Geometry check sheet. Reference: drawing and pictorial views, mm from the part's lowest x, y, z. A direction names the side the tool comes from. Round coordinates to 2 decimals unless told otherwise and drop trailing zeros. Write each loop counter-clockwise with the first axis right and the second up, starting at its lowest first coordinate (ties: lowest second). Pieces come first, ordered by that corner, then holes. Notation, with made-up numbers: (4, 69) -> (63, 69) arc R21 ccw to (63, 80) -> close; hole circle Ø8 at (39.5, 78.5). An arc over 180 degrees is marked (long way). Answer as a JSON object with one key per item and string values. Group by question number.
(1) Sectioned sample at D-D on z = 20.5. Record the cut outline in (x, y).
(2) Sectioned sample at A-A on x = 18.5. Record the cut outline in (y, z).
(3) Gauge pin test, flat ends, axial feed: pin 1 Ø5 at (y, z) = (3, 16.5) entering from -X; pin 2 Ø6 at (x, y) = (7.5, 7.5) entering from -Z; pin 3 Ø4 at (y, z) = (3.5, 3.5) entering from -X. Record the tip position at first contact, or that the pin passes through.
(4) Sectioned sample at B-B on z = 6.5. Record the cut outline in (x, y).
(5) Scan lines: L1, parallel to X at y = 5.75, z = 18.5; L2, parallel to Z at x = 9.75, y = 0.75; L3, parallel to Z at x = 17.75, y = 0.5. Record each from-to range of solid material in increasing order. Write a range as from..to.
(6) Draft check along X on the marked faces 1, 2, 3 and 4. Enter one of: released by +X, released by -X, zero draft, split by the parting line, or undercut.
(7) Set-up check for the marked faces 5 and 6: record each of +Z, -Z, +X, -X, +Y, -Y from which the full face is reachable in a straight line by a thin tool's end or side.
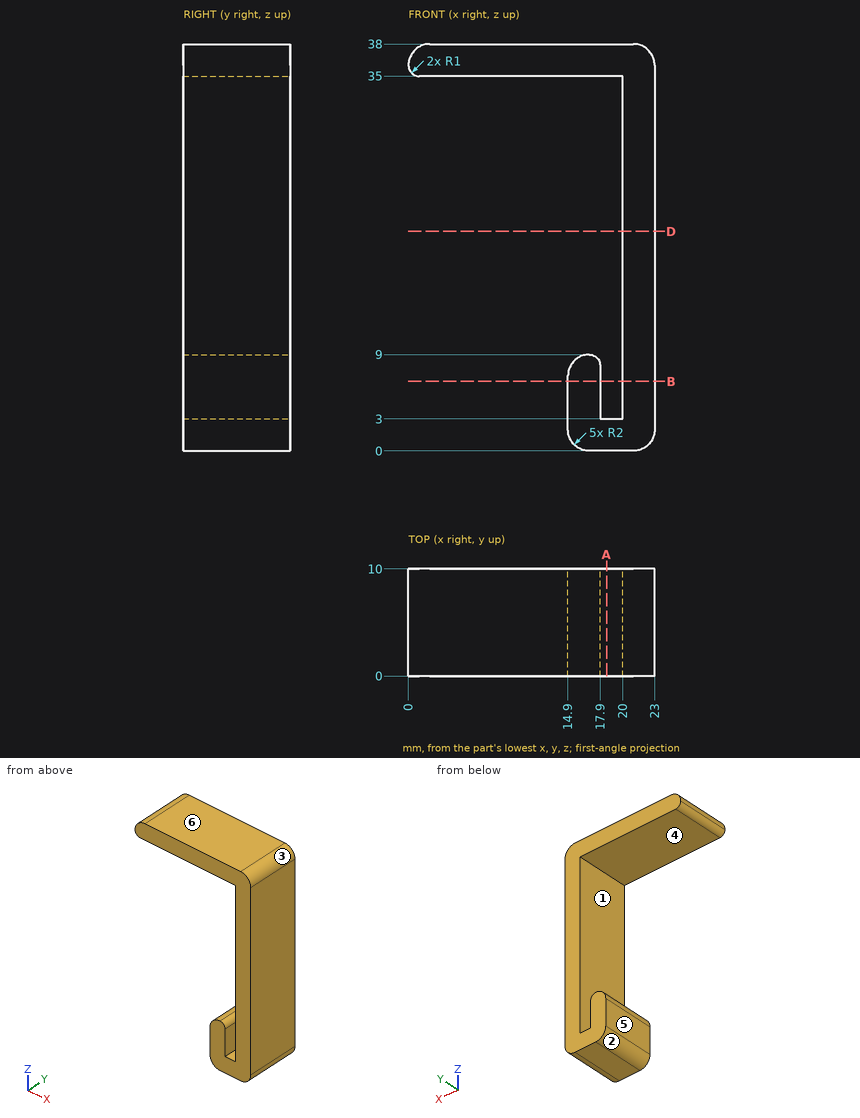
Computed values:
{
 "1": {"outline": "(20, 0) -> (23, 0) -> (23, 10) -> (20, 10) -> close"},
 "2": {"outline": "(0, 0) -> (10, 0) -> (10, 3) -> (0, 3) -> close; (0, 35) -> (10, 35) -> (10, 38) -> (0, 38) -> close"},
 "3": {"pin 1": "x = 20", "pin 2": "z = 35", "pin 3": "x = 14.9"},
 "4": {"outline": "(14.9, 0) -> (17.9, 0) -> (17.9, 10) -> (14.9, 10) -> close; (20, 0) -> (23, 0) -> (23, 10) -> (20, 10) -> close"},
 "5": {"L1": "20..23", "L2": "35..38", "L3": "0..8.53, 35..38"},
 "6": {"face 1": "undercut", "face 2": "released by -X", "face 3": "released by +X", "face 4": "zero draft"},
 "7": {"face 5": "-Z, -X, +Y, -Y", "face 6": "+Z, +X, -X, +Y, -Y"}
}
